For this review, take the finished solid that the model builds, in its own axes (mm). Round coordinates to 2 decimals unless told otherwise and drop trailing zeros. Order: outer loops, then holes, each group sorted by start corner. A loop starts at its lowest first (then second) coordinate and runs counter-clockwise, first axis right, second up. Notation, with made-up numbers: M 22,-28 L 48,-28 A21 cw 48,-13 Z; hole C 38,-38.5 d4. An arc over 180 degrees is marked long. Use a Markdown table: item, result.
Autodesk Inventor part; units mm, degrees
ref_plane "YZ Plane" through (0, 0, 0) normal (1, 0, 0) x (0, 1, 0)
ref_plane "XZ Plane" through (0, 0, 0) normal (0, 1, 0) x (-1, 0, 0)
ref_plane "XY Plane" through (0, 0, 0) normal (0, 0, 1) x (1, 0, 0)
sketch "Sketch1" plane through (0, 0, 0) normal (0, 0, 1) x (1, 0, 0)
  circle A0 centre (0, 0) radius 3.75
  circle A1 centre (0, 0) radius 3.5
  point P0 (0, 0)
  dimension "d0" = 7
extrude "Extrusion1" add sketch "Sketch1" along normal blind 3 contours A1
sketch "Sketch2" plane through (0, 0, 3) normal (0, 0, 1) x (1, 0, 0)
  circle A0 centre (0, 0) radius 3.05
  dimension "d3" = 6.1
extrude "Extrusion2" cut sketch "Sketch2" against normal blind 2.2
sketch "Sketch3" plane through (0, 0, 0.8) normal (0, 0, 1) x (1, 0, 0)
  circle A0 centre (0, 0) radius 0.75
  dimension "d6" = 1.5
extrude "Extrusion3" cut sketch "Sketch3" against normal blind 2.2
chamfer "Chamfer1" distance 0.5 angle 45 1 edges at (-3.5, 0, 0)
properties part number "ma_holder_1"
Q1. Clearance check with flat-ended pins moving along their axes: pin 1 (2 mm diameter, centred on x = 0, y = 0, fed in from +Z); pin 2 (1 mm diameter, centred on x = 1.5, z = 2, fed in from -Y). State where each tip first meets the part, or that it passes through.
Determined:
| item | result |
|---|---|
| pin 1 | stops at z = 0.8 |
| pin 2 | stops at y = -3.35 |
Q2. Draft analysis for pull direction Y (two halves, no side actions). For faces 1 (the cylindrical face through (-0.75, 0.03, 0.41)), 2 (the cylindrical face through (3.233, 1.341, 1.732)), 3 (the flat face through (1, -1, 0)), state which applies: pulls with the +Y half, pulls with the -Y half, needs draft (parallel to the pull), parting line crosses it, or undercut.
Determined:
| item | result |
|---|---|
| face 1 | undercut |
| face 2 | parting line crosses it |
| face 3 | needs draft |
Q3. Add section C-C (z = 1.2). Write out the cut boundary in (x, y).
Determined:
| item | result |
|---|---|
| outline | C 0,0 d7; hole C 0,0 d6.1 |
Q4. Wall thickness on line 1 along Y through (x, z) = (0, 1.7); line 2 along Y through (x, z) = (0, 0.65); line 3 along X through (y, z) = (2.5, 1.75): over which ranges is each line inside the solid? List them lowest first. Write a range as [from, to].
Determined:
| item | result |
|---|---|
| line 1 | y = [-3.5, -3.05], [3.05, 3.5] |
| line 2 | y = [-3.5, -0.75], [0.75, 3.5] |
| line 3 | x = [-2.45, -1.75], [1.75, 2.45] |
Q5. Add section A-A (y = 0). Write out the cut boundary in (x, z).
Determined:
| item | result |
|---|---|
| outline | M -3.5,0.5 L -3,0 L -0.75,0 L -0.75,0.8 L -3.05,0.8 L -3.05,3 L -3.5,3 Z; M 0.75,0 L 3,0 L 3.5,0.5 L 3.5,3 L 3.05,3 L 3.05,0.8 L 0.75,0.8 Z |
